```python
from build123d import *

# Parameters (mm, degrees)
PANEL_PROFILE_2_W       = 355.6
PANEL_PROFILE_2_H       = 203.2
PANEL_PROFILE_DEPTH     = 3.175
SKETCH8_R               = 1.8288
CUT_EXTRUDE1_DEPTH      = 10
FILLET1_R               = 6.35
CUT_EXTRUDE2_START      = -4.175
SKETCH9_W               = 38.18
SKETCH9_H               = 3.25
CUT_EXTRUDE2_DEPTH      = 5.175
MIRROR2_START           = -4.175
MIRROR2_COPY_1_SKETCH_W = 38.18
MIRROR2_COPY_1_SKETCH_H = 3.25
MIRROR2_COPY_1_DEPTH    = 5.175
CUT_EXTRUDE3_START      = -4.175
SKETCH10_W              = 3.2512
SKETCH10_H              = 38.1762
CUT_EXTRUDE3_DEPTH      = 5.175
MIRROR4_START           = -4.175
MIRROR4_COPY_1_SKETCH_W = 3.2512
MIRROR4_COPY_1_SKETCH_H = 38.1762
MIRROR4_COPY_1_DEPTH    = 5.175


with BuildPart() as part:
    # Panel Profile 2 → Panel-Profile (new body)
    with BuildSketch(Plane(origin=(0, 0, 0), x_dir=(1, 0, 0), z_dir=(0, 1, 0))):
        Rectangle(PANEL_PROFILE_2_W, PANEL_PROFILE_2_H)
    extrude(amount=-PANEL_PROFILE_DEPTH)

    # Sketch8 → Cut-Extrude1 (cut)
    with BuildSketch(Plane(origin=(0, 0, 0), x_dir=(1, 0, 0), z_dir=(0, 1, 0))):
        with Locations((-158.75, 82.55)):
            Circle(SKETCH8_R)
        with Locations((0, 82.55)):
            Circle(SKETCH8_R)
        with Locations((158.75, 82.55)):
            Circle(SKETCH8_R)
        with Locations((-158.75, -82.55)):
            Circle(SKETCH8_R)
        with Locations((0, -82.55)):
            Circle(SKETCH8_R)
        with Locations((158.75, -82.55)):
            Circle(SKETCH8_R)
    extrude(amount=-CUT_EXTRUDE1_DEPTH, mode=Mode.SUBTRACT)

    # Fillet1
    fillet1_edges = [part.edges().sort_by_distance(p)[0] for p in [
        (177.8, -1.5875, 101.6),
        (-177.8, -1.5875, 101.6),
        (-177.8, -1.5875, -101.6),
        (177.8, -1.5875, -101.6),
    ]]
    fillet(fillet1_edges, radius=FILLET1_R)

    # Sketch9 → Cut-Extrude2 (cut)
    with BuildSketch(Plane(origin=(0, 0, 0), x_dir=(1, 0, 0), z_dir=(0, 1, 0)).offset(CUT_EXTRUDE2_START)):
        with Locations((-127, 93.625)):
            Rectangle(SKETCH9_W, SKETCH9_H)
        with Locations((-50.8, 93.625)):
            Rectangle(SKETCH9_W, SKETCH9_H)
    cut_extrude2 = extrude(amount=CUT_EXTRUDE2_DEPTH, mode=Mode.SUBTRACT)

    # Mirror1: Cut-Extrude2 across plane
    add(cut_extrude2.mirror(Plane(origin=(0, 0, 0), x_dir=(0, 0, 1), z_dir=(1, 0, 0))), mode=Mode.SUBTRACT)

    # Mirror2: Cut-Extrude2 across plane
    add(cut_extrude2.mirror(Plane.XY), mode=Mode.SUBTRACT)

    # Mirror2 copy 1 sketch → Mirror2 copy 1 (cut)
    with BuildSketch(Plane(origin=(0, 0, 0), x_dir=(-1, 0, 0), z_dir=(0, 1, 0)).offset(MIRROR2_START)):
        with Locations((-127, 93.625)):
            Rectangle(MIRROR2_COPY_1_SKETCH_W, MIRROR2_COPY_1_SKETCH_H)
        with Locations((-50.8, 93.625)):
            Rectangle(MIRROR2_COPY_1_SKETCH_W, MIRROR2_COPY_1_SKETCH_H)
    extrude(amount=MIRROR2_COPY_1_DEPTH, mode=Mode.SUBTRACT)

    # Sketch10 → Cut-Extrude3 (cut)
    with BuildSketch(Plane(origin=(0, 0, 0), x_dir=(1, 0, 0), z_dir=(0, 1, 0)).offset(CUT_EXTRUDE3_START)):
        with Locations((-169.8244, 38.1)):
            Rectangle(SKETCH10_W, SKETCH10_H)
    cut_extrude3 = extrude(amount=CUT_EXTRUDE3_DEPTH, mode=Mode.SUBTRACT)

    # Mirror3: Cut-Extrude3 across plane
    add(cut_extrude3.mirror(Plane.XY), mode=Mode.SUBTRACT)

    # Mirror4: Cut-Extrude3 across plane
    add(cut_extrude3.mirror(Plane(origin=(0, 0, 0), x_dir=(0, 0, 1), z_dir=(1, 0, 0))), mode=Mode.SUBTRACT)

    # Mirror4 copy 1 sketch → Mirror4 copy 1 (cut)
    with BuildSketch(Plane(origin=(0, 0, 0), x_dir=(-1, 0, 0), z_dir=(0, 1, 0)).offset(MIRROR4_START)):
        with Locations((-169.8244, 38.1)):
            Rectangle(MIRROR4_COPY_1_SKETCH_W, MIRROR4_COPY_1_SKETCH_H)
    extrude(amount=MIRROR4_COPY_1_DEPTH, mode=Mode.SUBTRACT)


solid = part.part
```
Geometry: final body of the model. Coordinates: model frame, mm. Coordinates: 2 decimals unless noted, no trailing zeros. Loops run counter-clockwise (first coordinate to the right, second up) from the corner with the lowest first, then second, coordinate; pieces in that order, holes last. Notation, with made-up numbers: (56.5, 70.5) -> (114.5, 70.5) arc R27 cw to (114.5, 94.5) -> close; hole circle Ø2 at (-1.75, 82.25). An arc over 180 degrees is marked (long way). Use a Markdown table: item, result. Add a question column.
(1) Section query A-A, the plane x = -63. Return loops of the section in (y, z) (3 decimals).
(2) Line query: line 1 along X through (y, z) = (-1.6, 82.55); line 2 along Z through (x, y) = (-118.5, -1); line 3 along X through (y, z) = (-2.45, 37). Output: solid intervals per line, ascending.
(3) Section query B-B, the plane y = -2. State how many separate pieces and enclosed holes the cut face has, plus the area to 3 significant figures.
Answer:
| question | item | result |
|---|---|---|
| 1 | outline | (-3.175, -101.6) -> (0, -101.6) -> (0, -95.25) -> (-3.175, -95.25) -> close; (-3.175, -92) -> (0, -92) -> (0, 92) -> (-3.175, 92) -> close; (-3.175, 95.25) -> (0, 95.25) -> (0, 101.6) -> (-3.175, 101.6) -> close |
| 2 | line 1 | x = -177.8 to -160.58, -156.92 to -1.83, 1.83 to 156.92, 160.58 to 177.8 |
| 2 | line 2 | z = -101.6 to -95.25, -92 to 92, 95.25 to 101.6 |
| 2 | line 3 | x = -177.8 to -171.45, -168.2 to 168.2, 171.45 to 177.8 |
| 3 | separate pieces | 1 |
| 3 | enclosed holes | 18 |
| 3 | area | 70,700 mm^2 |
